Source: CAD feature listing. Evaluate the final solid. Frame: model axes, mm. A direction names the side the tool comes from. Round coordinates to 2 decimals unless told otherwise and drop trailing zeros. Order: outer loops, then holes, each group sorted by start corner. A loop starts at its lowest first (then second) coordinate and runs counter-clockwise, first axis right, second up. Notation, with made-up numbers: (80.25, -26) - (123.25, -26) arc R19 ccw to (123.25, 7) - close; hole circle Ø11 at (61.5, 70). An arc over 180 degrees is marked (long way). Return JSON: item names as keys, results as strings. Group by question number.
1) Section B-B, the plane y = 12.5. Return loops of the section in (x, z), plus the area to 3 significant figures.
2) Section A-A, the plane y = -1.5. Return loops of the section in (x, z).
3) Mould query, pull axis Z, two halves, no side actions, for faces 6 (the cylindrical face through (0, 6, -8)), 7 (the cylindrical face through (-9.76, 13.49, -2.17)), 8 (the flat face through (0, -3, -5.1)). Classes: pulls with the +Z half, pulls with the -Z half, needs draft (parallel to the pull), parting line crosses it, or undercut.
4) Access query for faces 1 (the flat face through (0, -3, 5.8)), 2 (the flat face through (-7.5, 6, 0)), 3 (the flat face through (7.5, 6, 0)), 4 (the flat face through (-6, 15, 3)), 5 (the cylindrical face through (0, 6, 8)). Directions: +Z, -Z, +X, -X, +Y, -Y. A direction counts if a zero-diameter tool reaches every point of the face in a straight line with its end or side. Return the directions, or none.
5) Ray query, line 1 (Z direction, x = 0.5, y = -0.5); line 2 (X direction, y = 8.5, z = -0.75); line 3 (Y direction, x = -5.25, z = -4.5). Return the intervals inside material, ascending. Write a range as from..to.
6) Contact query for flat-ended pins moving along their axis: P1, Ø2.5, axis at x = 0, y = -2, coming from the -Z side; P2, Ø10, axis at y = 3.5, z = -3.5, coming from the -X side; P3, Ø1.5, axis at x = 0.5, y = 11, coming from the +Z side. Output: stop coordinate, or through.
```python
from build123d import *

# Parameters (mm, degrees)
BOSS_EXTRUDE1_DEPTH = 13
SKETCH2_R           = 10
BOSS_EXTRUDE2_DEPTH = 2
CHAMFER1_SIZE       = 1
SKETCH3_R           = 6.5
BOSS_EXTRUDE3_DEPTH = 6.5
FILLET1_SIZE        = 2
FILLET1_SIZE_2      = 6.4
SKETCH4_W           = 3.2
SKETCH4_H           = 0.7
BOSS_EXTRUDE4_DEPTH = 5.3


with BuildPart() as part:
    # Sketch1 → Boss-Extrude1 (new body)
    with BuildSketch(Plane(origin=(0, 0, 0), x_dir=(1, 0, 0), z_dir=(0, 1, 0))):
        with BuildLine():
            Line((-7.5, 2.783882181), (-7.5, -2.783882181))
            ThreePointArc((-7.5, -2.783882181), (0, -8), (7.5, -2.783882181))
            Line((7.5, -2.783882181), (7.5, 2.783882181))
            ThreePointArc((7.5, 2.783882181), (0, 8), (-7.5, 2.783882181))
        make_face()
    extrude(amount=BOSS_EXTRUDE1_DEPTH)

    # Sketch2 → Boss-Extrude2 (add)
    with BuildSketch(Plane(origin=(0, 13, 0), x_dir=(1, 0, 0), z_dir=(0, 1, 0))):
        with Locations(Location((0, 0, 0), (0, 0, 270))):
            Circle(SKETCH2_R)
    extrude(amount=BOSS_EXTRUDE2_DEPTH)

    # Chamfer1
    chamfer1_edges = [part.edges().sort_by_distance(p)[0] for p in [
        (0, 15, -10),
    ]]
    chamfer(chamfer1_edges, length=CHAMFER1_SIZE)

    # Sketch3 → Boss-Extrude3 (add)
    with BuildSketch(Plane(origin=(0, 15, 0), x_dir=(1, 0, 0), z_dir=(0, 1, 0))):
        with Locations(Location((0, 0, 0), (0, 0, 90))):
            Circle(SKETCH3_R)
    extrude(amount=BOSS_EXTRUDE3_DEPTH)

    # Fillet1
    # an asymmetric fillet: 6.4, 2 mm, written as the material it takes off along each edge
    with BuildSketch(Plane(origin=(0, 21.5, 0), x_dir=(0, 0, -1), z_dir=(1, 0, 0))) as fillet1_piece_1:
        with BuildLine():
            Bezier((6.5, -FILLET1_SIZE), (6.5, 0), (6.5 - FILLET1_SIZE_2, 0), weights=[1, 0.707106781, 1])
            Line((6.5 - FILLET1_SIZE_2, 0), (6.5, 0))
            Line((6.5, 0), (6.5, -FILLET1_SIZE))
        make_face()
    revolve(axis=Axis((0, 21.5, 0), (0, 1, 0)), mode=Mode.SUBTRACT)

    # Sketch4 → Boss-Extrude4 (add)
    with BuildSketch(Plane.XZ):
        with Locations((0, 5.45)):
            Rectangle(SKETCH4_W, SKETCH4_H)
        with Locations((0, -5.45)):
            Rectangle(SKETCH4_W, SKETCH4_H)
    extrude(amount=BOSS_EXTRUDE4_DEPTH)


solid = part.part
```
Geometry check:
{
 "1": {"outline": "(-7.5, -2.78) arc R8 ccw to (7.5, -2.78) - (7.5, 2.78) arc R8 ccw to (-7.5, 2.78) - close", "area": "197 mm2"},
 "2": {"outline": "(-1.6, -5.8) - (1.6, -5.8) - (1.6, -5.1) - (-1.6, -5.1) - close; (-1.6, 5.1) - (1.6, 5.1) - (1.6, 5.8) - (-1.6, 5.8) - close"},
 "3": {"face 6": "pulls with the -Z half", "face 7": "parting line crosses it", "face 8": "undercut"},
 "4": {"face 1": "+Z, +X, -X, -Y", "face 2": "+Z, -Z, -X, -Y", "face 3": "+Z, -Z, +X, -Y", "face 4": "+Y", "face 5": "+Z, -Y"},
 "5": {"line 1": "-5.8..-5.1, 5.1..5.8", "line 2": "-7.5..7.5", "line 3": "0..15"},
 "6": {"P1": "z = -5.8", "P2": "x = -7.5", "P3": "z = 8"}
}
